Part model, mm, in its own coordinate system. A direction names the side the tool comes from. Round coordinates to 2 decimals unless told otherwise and drop trailing zeros. Write each loop counter-clockwise with the first axis right and the second up, starting at its lowest first coordinate (ties: lowest second). Pieces come first, ordered by that corner, then holes.
1) Saw through at B-B on z = -12.75. Write the cut outline in (x, y), and give its area (3 significant figures).
2) Flat gauge pins, fed straight in: pin 1 (1.4 mm diameter, centred on x = 12.5, z = -14, fed in from -Y); pin 2 (5 mm diameter, centred on y = 29.5, z = -6.5, fed in from -X). Where does each tip first touch, or does it go through?
3) Pull direction X, two halves, no side cores. Call faces 1 (the cylindrical face through (10.79, 2.46, -12.53)), 2 (the flat face through (1.398, 46.342, -16.126)), 3 (the flat face through (32, 0, -14)): +X half, -X half, draft (parallel to the pull), parting line (faces both ways), or undercut.
4) Saw through at A-A on y = 84. Write the cut outline in (x, z).
5) Drill centre lines: L1, parallel to X at y = 1.65, z = -14; L2, parallel to Z at x = 31.5, y = 41.5. Where is each one in solid material? Low to high.
6) Which spindle directions (+Z, -Z, +X, -X, +Y, -Y) get a long thin tool onto all of the face, cutting with end or side? Do faces 4 (the flat face through (34.48, 46.34, -1.49)), 5 (the flat face through (13, 5, -14)), 6 (the flat face through (63.562, 46.342, -16.068)), 7 (the flat face through (0, 46, -23)), 8 (the flat face through (1.438, 46.342, -11.932)). Say none if no direction does.
```python
from build123d import *

# Parameters (mm, degrees)
BOSS_EXTRUDE1_DEPTH = 94
SKETCH1_3_R         = 2.40784246
CUT_EXTRUDE1_DEPTH  = 5


with BuildPart() as part:
    # Sketch1 → Boss-Extrude1 (new body)
    with BuildSketch(Plane(origin=(0, 0, 0), x_dir=(1, 0, 0), z_dir=(0, 1, 0))):
        Polygon((0, 9.805763686), (0, 0), (28.48646363, 0), (32.5, 2.93900405), (36.51353637, 0), (65, 0), (65, 9.805763686), (62.163382508, 14), (65, 18.194236314), (65, 28), (0, 28), (0, 18.194236314), (2.836617492, 14), align=None)
    extrude(amount=BOSS_EXTRUDE1_DEPTH)

    # Sketch1<3> → Cut-Extrude1 (cut)
    with BuildSketch(Plane(origin=(0, 0, 0), x_dir=(1, 0, 0), z_dir=(0, 1, 0))):
        with Locations((12.697649227, 14)):
            Circle(SKETCH1_3_R)
    extrude(amount=CUT_EXTRUDE1_DEPTH, mode=Mode.SUBTRACT)


solid = part.part
```
Completed:
1. outline: (1.99, 0) - (10.64, 0) - (10.64, 5) - (14.76, 5) - (14.76, 0) - (63.01, 0) - (63.01, 94) - (1.99, 94) - close
1. area: 5,720 mm2
2. pin 1: stops at y = 5
2. pin 2: stops at x = 0
3. face 1: undercut
3. face 2: -X half
3. face 3: draft
4. outline: (0, -28) - (65, -28) - (65, -18.19) - (62.16, -14) - (65, -9.81) - (65, 0) - (36.51, 0) - (32.5, -2.94) - (28.49, 0) - (0, 0) - (0, -9.81) - (2.84, -14) - (0, -18.19) - close
5. L1: x = 2.84 to 10.29, 15.11 to 62.16
5. L2: z = -28 to -2.21
6. face 4: +Z, +Y, -Y
6. face 5: -Y
6. face 6: +X, +Y, -Y
6. face 7: +Z, -Z, -X, +Y, -Y
6. face 8: -X, +Y, -Y
